Could you check a few things on this model? Use its own coordinates, in mm. A direction names the side the tool comes from. Coordinates: 2 decimals unless noted, no trailing zeros. Order: outer loops, then holes, each group sorted by start corner. A loop starts at its lowest first (then second) coordinate and runs counter-clockwise, first axis right, second up. Notation, with made-up numbers: (24.5, 11.25) - (30.5, 11.25) arc R25 ccw to (30.5, 42.25) - close; hole circle Ø8 at (-22.75, 25). An arc over 180 degrees is marked (long way). One line per item, written item: value.
Autodesk Inventor part; units mm, degrees
ref_plane "XZ Plane" through (0, 0, 0) normal (0, 1, 0) x (-1, 0, 0)
ref_plane "XY Plane" through (0, 0, 0) normal (0, 0, 1) x (1, 0, 0)
sketch "Sketch1" plane through (0, 0, 0) normal (0, 1, 0) x (-1, 0, 0)
  circle A0 centre (0, 0) radius 1.1
  circle A1 centre (0, 0) radius 2.575
  dimension "d0" = 2.2
  dimension "d1" = 5.15
extrude "Extrusion1" add sketch "Sketch1" along normal blind 18
sketch "Sketch2" plane through (0, 0, 0) normal (0, 0, 1) x (1, 0, 0)
  line L0 (2.575, 18) -> (-2.575, 18)
  line L1 (2.575, 0) -> (-2.575, 0)
  line L2 (-2.575, 0) -> (-2.575, 18)
  line L3 (-2.575, 16) -> (2.5173, 16)
  line L4 (2.575, 18) -> (-2.575, 18)
  line L5 (0, 18) -> (0, 0)
  circle A0 centre (0, 14) radius 2
  dimension "d4" = 2
  dimension "d5" = 4
extrude "Extrusion2" cut sketch "Sketch2" along normal blind 12 contours A0 L5 | L5 A0
sketch "Sketch3" plane through (0, 0, 0) normal (1, 0, 0) x (0, 1, 0)
  line L0 (18, -2.575) -> (18, 2.575)
  line L1 (0, -2.575) -> (0, 2.575)
  line L2 (0, 2.575) -> (18, 2.575)
  line L3 (16, 2.575) -> (16, -2.525)
  line L4 (18, 1.1) -> (18, -1.1)
  line L5 (18, 0) -> (0, 0)
  circle A0 centre (14, 0) radius 2
  point P0 (14, 1.6219)
  dimension "d8" = 2
  dimension "d9" = 4
extrude "Extrusion3" cut sketch "Sketch3" along normal up to next contours A0 L5 | L5 A0
chamfer "Chamfer1" distance 0.2 angle 45 4 edges at (1.1, 0, 0) (2.575, 0, 0) (1.1, 18, 0) (2.575, 18, 0)
properties part number "motor_shaft_adapter"
Item 1: I want a section at A-A on y = 15.5. Please give me the cut outline in (x, z) (3 decimals), then the cut area to 3 significant figures.
Conclusion:
outline: (-1.323, 0) - (-1.323, 2.209) arc R2.575 ccw (long way) to (2.209, -1.323) - (0, -1.323) - (0, -1.1) arc R1.1 cw to (-1.1, 0) - close; (1.323, 1.323) - (2.209, 1.323) arc R2.575 ccw to (1.323, 2.209) - close
area: 8.63 mm²
Item 2: If I drill on probe 1 along X at (y, z) = (6.25, 0) (3 decimals); probe 2 along Y at (x, z) = (-0.4, 1.1), over which ranges is the centre line in solid material (lowest first)?
Conclusion:
probe 1: -2.575 to -1.1, 1.1 to 2.575
probe 2: 0.13 to 12.04, 15.96 to 17.87
Item 3: I'm going to push flat-ended pins straight in: pin 1 Ø2 at (x, z) = (0, 0) entering from +Y; pin 2 Ø0.7 at (x, y) = (-1.5, 14.5) entering from +Z; pin 3 Ø0.7 at (y, z) = (14.5, -1.5) entering from +X. Where does each tip first touch, or does it pass through?
Conclusion:
pin 1: through
pin 2: z = 0
pin 3: x = 0
Item 4: Thinking about a two-plate mould opening in Y: for faces 4 (the face through (0, 14, -1.4)), 5 (the face through (-1.05, 6.92, -0.33)), 6 (the face through (0, 0, -2)), 7 (the face through (-2, 14, 1)), which applies, pulls with the +Y half, pulls with the -Y half, needs draft (parallel to the pull), parting line crosses it, or undercut?
Conclusion:
face 4: undercut
face 5: needs draft
face 6: pulls with the -Y half
face 7: undercut
Item 5: I want a section at D-D on y = 6.5. Please give me the cut outline in (x, z) (3 decimals), then the cut area to 3 significant figures.
Conclusion:
outline: circle Ø5.15 at (0, 0); hole circle Ø2.2 at (0, 0)
area: 17.0 mm²
Item 6: For faces 1 (the face through (-1.384, 8.877, -2.171)), 2 (the face through (-1.5, 14, 0)), 3 (the face through (1, 14, -2)), which set-ups out of +Z, -Z, +X, -X, +Y, -Y let a thin tool reach every point of the face, with its end or its side?
Conclusion:
face 1: +Y, -Y
face 2: +Z, +X
face 3: +X
Item 7: I want a section at B-B on z = 0.4. Give the number of separate pieces and of enclosed holes in the cut face, then the cut area to 3 significant figures.
Conclusion:
separate pieces: 3
enclosed holes: 0
area: 46.2 mm²
